Can you work these out from the model? Positions are in its coordinate system, mm. Give positions to 0.01 mm unless a question says otherwise; leave off trailing zeros. Order: outer loops, then holes, each group sorted by start corner. A loop starts at its lowest first (then second) coordinate and runs counter-clockwise, first axis right, second up. Notation, with made-up numbers: M -35,16.25 L -15,16.25 A17 ccw -15,26.25 Z; hole C -33,40 d2. An arc over 180 degrees is marked long. Answer as a JSON object with one key per item and string values.
```python
from build123d import *

# Parameters (mm, degrees)
F0_R     = 11.0109
F1_DEPTH = 6.35
F3_DEPTH = 6.35


with BuildPart() as f1:
    # F0 (on Top) → F1 (new body)
    with BuildSketch(Plane.XY):
        with BuildLine():
            ThreePointArc((-12.6025190653, 8.6339348228), (-40.3705251806, 10.8193243169), (-13.2862595435, 4.3169673779))
            ThreePointArc((-13.2862595435, 4.3169673779), (-12.7745129499, 6.4485453288), (-12.6025190653, 8.6339348228))
        make_face()
        with Locations((-26.5725190653, 8.6339348228)):
            Circle(F0_R, mode=Mode.SUBTRACT)
    extrude(amount=F1_DEPTH)



with BuildPart() as f1b:
    # F0 (on Top) → F1, piece 2 (new body)
    with BuildSketch(Plane.XY):
        with BuildLine():
            ThreePointArc((13.97, 27.94), (-9.8782817326, 37.8182817338), (-1.8e-09, 13.97))
            ThreePointArc((-1.8e-09, 13.97), (9.8782817326, 18.0617182662), (13.97, 27.94))
        make_face()
        with BuildLine():
            ThreePointArc((11.0109, 27.94), (7.785882057, 20.154117943), (0, 16.9291))
            ThreePointArc((0, 16.9291), (-7.785882057, 35.725882057), (11.0109, 27.94))
        make_face(mode=Mode.SUBTRACT)
    extrude(amount=F1_DEPTH)


with BuildPart() as f1c:
    # F0 (on Top) → F1, piece 3 (new body)
    with BuildSketch(Plane.XY):
        with BuildLine():
            ThreePointArc((40.5425190653, 8.6339348228), (24.387129585, 22.4319409404), (13.2862595349, 4.3169674044))
            ThreePointArc((13.2862595349, 4.3169674044), (28.7579085455, -5.1640712947), (40.5425190653, 8.6339348228))
        make_face()
        with Locations((26.5725190653, 8.6339348228)):
            Circle(F0_R, mode=Mode.SUBTRACT)
    extrude(amount=F1_DEPTH)


with BuildPart() as f1d:
    # F0 (on Top) → F1, piece 4 (new body)
    with BuildSketch(Plane.XY):
        with BuildLine():
            ThreePointArc((30.3927199491, -22.6039348228), (22.7649672257, -10.1565736775), (8.2113599659, -11.3019674177))
            ThreePointArc((8.2113599659, -11.3019674177), (10.0804726724, -35.0512959682), (30.3927199491, -22.6039348228))
        make_face()
        with Locations((16.4227199491, -22.6039348228)):
            Circle(F0_R, mode=Mode.SUBTRACT)
    extrude(amount=F1_DEPTH)


with BuildPart() as f1e:
    # F0 (on Top) → F1, piece 5 (new body)
    with BuildSketch(Plane.XY):
        with BuildLine():
            ThreePointArc((-2.4527199491, -22.6039348228), (-3.9753588409, -16.2616874733), (-8.2113600984, -11.3019673214))
            ThreePointArc((-8.2113600984, -11.3019673214), (-28.8700810572, -28.9461821724), (-2.4527199491, -22.6039348228))
        make_face()
        with Locations((-16.4227199491, -22.6039348228)):
            Circle(F0_R, mode=Mode.SUBTRACT)
    extrude(amount=F1_DEPTH)


with BuildPart() as f1f:
    # F0 (on Top) → F1, piece 6 (new body)
    with BuildSketch(Plane.XY):
        with BuildLine():
            ThreePointArc((13.2862595349, 4.3169674044), (8.2113599768, 11.3019674098), (-1.8e-09, 13.97))
            ThreePointArc((-1.8e-09, 13.97), (-8.2113599895, 11.3019674005), (-13.2862595435, 4.3169673779))
            ThreePointArc((-13.2862595435, 4.3169673779), (-13.2862595509, -4.3169673554), (-8.2113600984, -11.3019673214))
            ThreePointArc((-8.2113600984, -11.3019673214), (-8.19e-08, -13.97), (8.2113599659, -11.3019674177))
            ThreePointArc((8.2113599659, -11.3019674177), (12.4473611405, -6.3422472861), (13.97, 0))
            ThreePointArc((13.97, 0), (13.7980061187, 2.185389473), (13.2862595349, 4.3169674044))
        make_face()
        with BuildLine():
            ThreePointArc((0, 11.0109), (7.785882057, 7.785882057), (11.0109, 0))
            ThreePointArc((11.0109, 0), (-7.785882057, -7.785882057), (0, 11.0109))
        make_face(mode=Mode.SUBTRACT)
    extrude(amount=F1_DEPTH)


with BuildPart() as f1_1:
    add(f1.part)

    add(f1b.part)  # F3 merges F1b

    add(f1c.part)  # F3 merges F1c

    add(f1d.part)  # F3 merges F1d

    add(f1e.part)  # F3 merges F1e

    add(f1f.part)  # F3 merges F1f
    # F2 (on face) → F3 (join)
    with BuildSketch(Plane(origin=(0, 0, 0), x_dir=(1, 0, 0), z_dir=(0, 0, -1))):
        with BuildLine():
            ThreePointArc((2.4527199491, 22.6039348228), (0, 20.4182749221), (-2.4527199491, 22.6039348228))
            ThreePointArc((-2.4527199491, 22.6039348228), (-3.9753588004, 16.2616875527), (-8.2113599542, 11.3019674262))
            ThreePointArc((-8.2113599542, 11.3019674262), (-1.7e-08, 13.97), (8.2113599266, 11.3019674462))
            ThreePointArc((8.2113599266, 11.3019674462), (3.9753587927, 16.2616875678), (2.4527199491, 22.6039348228))
        make_face()
        with BuildLine():
            ThreePointArc((-8.2113599542, 11.3019674262), (-14.23733046, 8.8059287067), (-20.7396873605, 9.3176752902))
            ThreePointArc((-20.7396873605, 9.3176752902), (-19.4189334161, 6.3095939467), (-22.2555516539, 4.6523247098))
            ThreePointArc((-22.2555516539, 4.6523247098), (-16.6942373027, 1.2443468809), (-13.286259507, -4.3169674905))
            ThreePointArc((-13.286259507, -4.3169674905), (-13.2862595416, 4.3169673838), (-8.2113599542, 11.3019674262))
        make_face()
        with BuildLine():
            ThreePointArc((-7.22e-08, -13.97), (-8.2113599701, -11.3019674146), (-13.286259507, -4.3169674905))
            ThreePointArc((-13.286259507, -4.3169674905), (-12.7745129407, -6.4485453873), (-12.6025190653, -8.6339348228))
            ThreePointArc((-12.6025190653, -8.6339348228), (-13.2862595326, -12.9509022343), (-15.2705516539, -16.8452947974))
            ThreePointArc((-15.2705516539, -16.8452947974), (-12.0015608764, -16.5187314078), (-11.3019674114, -19.7286400255))
            ThreePointArc((-11.3019674114, -19.7286400255), (-6.3422473135, -15.4926388735), (-7.22e-08, -13.97))
        make_face()
        with BuildLine():
            ThreePointArc((13.2862595349, -4.3169674044), (8.2113599483, -11.3019674305), (-7.22e-08, -13.97))
            ThreePointArc((-7.22e-08, -13.97), (6.3422472492, -15.4926388407), (11.3019674114, -19.7286400255))
            ThreePointArc((11.3019674114, -19.7286400255), (12.0015608764, -16.5187314078), (15.2705516539, -16.8452947974))
            ThreePointArc((15.2705516539, -16.8452947974), (12.7745129466, -10.8193242958), (13.2862595349, -4.3169674044))
        make_face()
        with BuildLine():
            ThreePointArc((20.7396873605, 9.3176752902), (14.2373304432, 8.8059287094), (8.2113599266, 11.3019674462))
            ThreePointArc((8.2113599266, 11.3019674462), (12.4473611295, 6.3422473077), (13.97, 0))
            ThreePointArc((13.97, 0), (13.7980061187, -2.185389473), (13.2862595349, -4.3169674044))
            ThreePointArc((13.2862595349, -4.3169674044), (16.6942373347, 1.2443469129), (22.2555516539, 4.6523247098))
            ThreePointArc((22.2555516539, 4.6523247098), (19.4189334161, 6.3095939467), (20.7396873605, 9.3176752902))
        make_face()
    extrude(amount=-F3_DEPTH)


solid = f1_1.part
```
1) I'm going to push flat-ended pins straight in: pin 1 Ø17.5 at (x, y) = (26.57, 8.63) entering from -Z; pin 2 Ø1 at (y, z) = (-21, 1.5) entering from +X. Where does each tip first touch, or does it pass through?
Results found:
{"pin 1": "passes through", "pin 2": "stops at x = 30.35"}
2) I want a section at A-A on y = -26. Write out the boundary of the cut face in (x, z), and give its area (3 significant figures).
Results found:
{"outline": "M -29.97,0 L -26.9,0 L -26.9,6.35 L -29.97,6.35 Z; M -5.95,0 L -2.87,0 L -2.87,6.35 L -5.95,6.35 Z; M 2.87,0 L 5.95,0 L 5.95,6.35 L 2.87,6.35 Z; M 26.9,0 L 29.97,0 L 29.97,6.35 L 26.9,6.35 Z", "area": "78.2 mm²"}
3) I want a section at C-C on y = 31.5. Write out the boundary of the cut face in (x, z).
Results found:
{"outline": "M -13.51,0 L -10.42,0 L -10.42,6.35 L -13.51,6.35 Z; M 10.42,0 L 13.51,0 L 13.51,6.35 L 10.42,6.35 Z"}
4) Thinking about a two-plate mould opening in Y: for faces 1 (the face through (0.05, -20.42, 3.13)), 2 (the face through (-20.653, 17.918, 3.131)), 3 (the face through (-0.2, 11.2, 0)), which applies, pulls with the +Y half, pulls with the -Y half, needs draft (parallel to the pull), parting line crosses it, or undercut?
Results found:
{"face 1": "pulls with the -Y half", "face 2": "undercut", "face 3": "needs draft"}
5) I need wall thicknesses on L1, parallel to X at y = 0, z = 4.5; L2, parallel to X at y = 13, z = 5.75; L3, parallel to X at y = 8.5, z = 5.75. Which ranges of each line are inside material? Lowest first, please.
Results found:
{"L1": "x = -37.56 to -33.41, -19.74 to -11.01, 11.01 to 19.74, 33.41 to 37.56", "L2": "x = -39.84 to -36.68, -16.46 to 16.46, 36.68 to 39.84", "L3": "x = -40.54 to -37.58, -15.56 to -7, 7 to 15.56, 37.58 to 40.54"}
6) I want a section at D-D on y = -17. Write out the boundary of the cut face in (x, z), and give its area (3 significant figures).
Results found:
{"outline": "M -29.22,0 L -25.9,0 L -25.9,6.35 L -29.22,6.35 Z; M -6.94,0 L 6.94,0 L 6.94,6.35 L -6.94,6.35 Z; M 25.9,0 L 29.22,0 L 29.22,6.35 L 25.9,6.35 Z", "area": "130 mm²"}
7) I want a section at B-B on z = 2.5. Write out the boundary of the cut face in (x, y), and give its area (3 significant figures).
Results found:
{"outline": "M -22.26,-4.65 A2.47 cw -20.74,-9.32 A13.97 ccw long -2.45,-22.6 A2.47 cw 2.45,-22.6 A13.97 ccw long 20.74,-9.32 A2.47 cw 22.26,-4.65 A13.97 ccw long 15.27,16.85 A2.47 cw 11.3,19.73 A13.97 ccw long -11.3,19.73 A2.47 cw -15.27,16.85 A13.97 ccw long Z; hole C -26.57,8.63 d22.02; hole C -16.42,-22.6 d22.02; hole C 0,0 d22.02; hole C 0,27.94 d22.02; hole C 16.42,-22.6 d22.02; hole C 26.57,8.63 d22.02", "area": "1,680 mm²"}
